Here's how the part is built. I have some questions about the finished solid (model axes, mm). Face numbers are marked on the shaded views. A direction names the side the tool comes from. Coordinates: 2 decimals unless noted, no trailing zeros. Write each loop counter-clockwise with the first axis right and the second up, starting at its lowest first coordinate (ties: lowest second). Pieces come first, ordered by that corner, then holes.
Item 1: I want a section at B-B (z = -7.5). Please give me the cut outline in (x, y).
Item 2: For the marked faces 1 and 2, which set-ups out of +Z, -Z, +X, -X, +Y, -Y let a thin tool reach every point of the face, with its end or its side?
Item 3: I want a section at C-C (y = -12.5). Please give me the cut outline in (x, z).
Item 4: I'm going to push flat-ended pins straight in: P1, Ø7.5, axis at x = 42, y = -17.5, coming from the -Z side; P2, Ø5, axis at y = -10, z = -6.5, coming from the -X side. Where does each tip first touch, or does it pass through?
Item 5: Please list where these lines run through material, in increasing order: line 1 (Z direction, x = 74.4, y = -12.5); line 2 (Z direction, x = 64, y = -20); line 3 (Z direction, x = 74.5, y = -11).
Item 6: I want a section at A-A (y = -20). Please give me the cut outline in (x, z), and give its area (3 significant figures).
Item 7: I want a section at D-D (x = 67.5). Please give me the cut outline in (y, z), and give its area (3 significant figures).
from build123d import *

# Parameters (mm, degrees)
F0_W     = 6
F0_H     = 2
F0_W_2   = 20
F0_H_2   = 5
F1_DEPTH = 25
F2_R     = 2.5
F3_DEPTH = 20.001
F4_R     = 2
F5_DEPTH = 6
F6_SIZE  = 2


with BuildPart() as f1:
    # F0 (on Front) → F1 (new body)
    with BuildSketch(Plane.XZ):
        with Locations((74.487355, 1.5)):
            Rectangle(F0_W, F0_H)
        Polygon((2.951456, 12.5), (-0.512645, 10.5), (77.487355, 10.5), (77.487355, 12.5), align=None)
        with Locations((67.487355, -10)):
            Rectangle(F0_W_2, F0_H_2)
        with Locations((74.487355, 3.5)):
            Rectangle(F0_W, F0_H)
        Polygon((77.487355, 10.5), (-0.512645, 10.5), (-0.512645, -2.5), (57.487355, -2.5), (57.487355, -7.5), (77.487355, -7.5), (77.487355, 0.5), (71.487355, 0.5), (70.332654, 2.5), (71.487355, 4.5), (77.487355, 4.5), align=None)
        Polygon((71.487355, 2.5), (70.332654, 2.5), (71.487355, 0.5), align=None)
        Polygon((71.487355, 2.5), (71.487355, 4.5), (70.332654, 2.5), align=None)
    extrude(amount=F1_DEPTH)

    # F2 (on face) → F3 (cut, through all)
    with BuildSketch(Plane(origin=(57.487355, 0, 0), x_dir=(0, -1, 0), z_dir=(-1, 0, 0))):
        with Locations((20, -7.5)):
            Circle(F2_R)
        with Locations((5, -7.5)):
            Circle(F2_R)
    extrude(amount=-F3_DEPTH, mode=Mode.SUBTRACT)

    # F4 (on face) → F5 (cut)
    with BuildSketch(Plane.YZ.offset(77.487355)):
        with Locations((-12.5, 2.5)):
            Circle(F4_R)
        with Locations((-12.5, -7.5)):
            Circle(F4_R)
    extrude(amount=-F5_DEPTH, mode=Mode.SUBTRACT)

    # F6
    f6_edges = [f1.edges().sort_by_distance(p)[0] for p in [
        (40.219405, -25, 12.5),
    ]]
    chamfer(f6_edges, length=F6_SIZE)


solid = f1.part
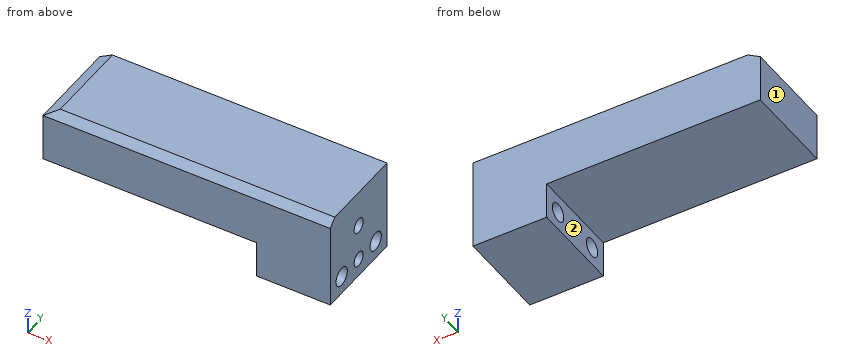
Answer:
1. outline: (57.49, -25) - (77.49, -25) - (77.49, -22.5) - (57.49, -22.5) - close; (57.49, -17.5) - (77.49, -17.5) - (77.49, -14.5) - (71.49, -14.5) - (71.49, -10.5) - (77.49, -10.5) - (77.49, -7.5) - (57.49, -7.5) - close; (57.49, -2.5) - (77.49, -2.5) - (77.49, 0) - (57.49, 0) - close
2. face 1: +Z, -Z, -X, +Y, -Y
2. face 2: -Z, -X, +Y, -Y
3. outline: (-0.51, -2.5) - (57.49, -2.5) - (57.49, -12.5) - (77.49, -12.5) - (77.49, -9.5) - (71.49, -9.5) - (71.49, -5.5) - (77.49, -5.5) - (77.49, 0.5) - (71.49, 0.5) - (71.49, 4.5) - (77.49, 4.5) - (77.49, 12.5) - (2.95, 12.5) - (-0.51, 10.5) - close
4. P1: stops at z = -2.5
4. P2: stops at x = 57.49
5. line 1: z = -12.5 to -9.5, -5.5 to 0.5, 4.5 to 12.5
5. line 2: z = -12.5 to -10, -5 to 12.5
5. line 3: z = -12.5 to -8.82, -6.18 to 1.18, 3.82 to 12.5
6. outline: (-0.51, -2.5) - (57.49, -2.5) - (57.49, -5) - (77.49, -5) - (77.49, 12.5) - (2.95, 12.5) - (-0.51, 10.5) - close; (57.49, -12.5) - (77.49, -12.5) - (77.49, -10) - (57.49, -10) - close
6. area: 1,270 mm2
7. outline: (-25, -12.5) - (0, -12.5) - (0, 12.5) - (-23, 12.5) - (-25, 10.5) - close; hole circle Ø5 at (-20, -7.5); hole circle Ø5 at (-5, -7.5)
7. area: 584 mm2
